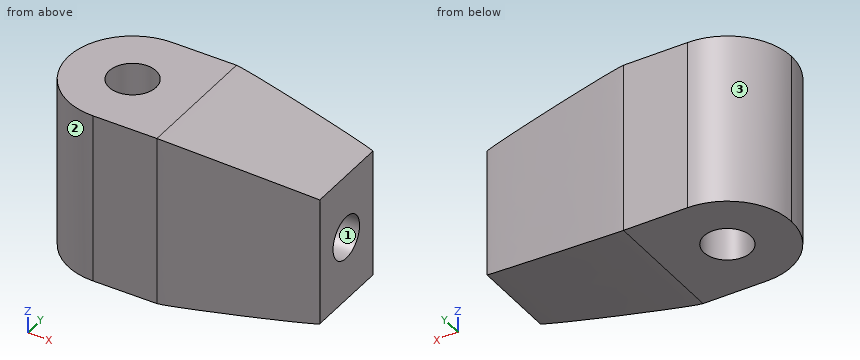
from build123d import *

# Parameters (mm, degrees)
SKETCH_1_W          = 13
SKETCH_1_H          = 8
EXTRUDE_1_DEPTH     = 6
SKETCH_2_R          = 1.1
CUT_EXTRUDE_1_DEPTH = 17.401219467
SKETCH_3_R          = 1
CUT_EXTRUDE_2_DEPTH = 8
FILLET_1_SIZE       = 1
FILLET_1_SIZE_2     = 7
FILLET_2_R          = 3


# Some blends are built 0.0001 mm under size
with BuildPart() as part:
    # 草图1 → 凸台-拉伸1 (new body)
    with BuildSketch(Plane(origin=(0, 0, 0), x_dir=(1, 0, 0), z_dir=(0, 1, 0))):
        with Locations((6.5, 4)):
            Rectangle(SKETCH_1_W, SKETCH_1_H)
    extrude(amount=EXTRUDE_1_DEPTH)

    # 草图2 → 切除-拉伸1 (cut, through all)
    with BuildSketch(Plane.XY):
        with Locations((3, 3)):
            Circle(SKETCH_2_R)
    extrude(amount=-CUT_EXTRUDE_1_DEPTH, mode=Mode.SUBTRACT)

    # 草图3 → 切除-拉伸2 (cut)
    with BuildSketch(Plane(origin=(13, 0, 0), x_dir=(0, 0, -1), z_dir=(1, 0, 0))):
        with Locations((4, 3)):
            Circle(SKETCH_3_R)
    extrude(amount=-CUT_EXTRUDE_2_DEPTH, mode=Mode.SUBTRACT)

    # 圆角1
    # a fillet whose section is not a circle: 7, 1 mm, written as the material it takes off along each edge
    with BuildSketch(Plane(origin=(13, -17.5, -8), x_dir=(0, 0, 1), z_dir=(0, 1, 0))) as fillet_1_piece_1:
        with BuildLine():
            Bezier((FILLET_1_SIZE, 0), (0, 0), (0, -FILLET_1_SIZE_2), weights=[1, 0.052631579, 1])
            Line((0, -FILLET_1_SIZE_2), (0, 0))
            Line((0, 0), (FILLET_1_SIZE, 0))
        make_face()
    extrude(amount=41, mode=Mode.SUBTRACT)
    with BuildSketch(Plane(origin=(13, 0, 17.5), x_dir=(-1, 0, 0), z_dir=(0, 0, -1))) as fillet_1_piece_2:
        with BuildLine():
            Bezier((FILLET_1_SIZE_2, 0), (0, 0), (0, FILLET_1_SIZE), weights=[1, 0.052631579, 1])
            Line((0, FILLET_1_SIZE), (0, 0))
            Line((0, 0), (FILLET_1_SIZE_2, 0))
        make_face()
    extrude(amount=43, mode=Mode.SUBTRACT)
    with BuildSketch(Plane(origin=(13, -17.5, 0), x_dir=(-1, 0, 0), z_dir=(0, 1, 0))) as fillet_1_piece_3:
        with BuildLine():
            Bezier((FILLET_1_SIZE_2, 0), (0, 0), (0, -FILLET_1_SIZE), weights=[1, 0.052631579, 1])
            Line((0, -FILLET_1_SIZE), (0, 0))
            Line((0, 0), (FILLET_1_SIZE_2, 0))
        make_face()
    extrude(amount=41, mode=Mode.SUBTRACT)
    with BuildSketch(Plane(origin=(13, 6, 17.5), x_dir=(-1, 0, 0), z_dir=(0, 0, -1))) as fillet_1_piece_4:
        with BuildLine():
            Bezier((FILLET_1_SIZE_2, 0), (0, 0), (0, -FILLET_1_SIZE), weights=[1, 0.052631579, 1])
            Line((0, -FILLET_1_SIZE), (0, 0))
            Line((0, 0), (FILLET_1_SIZE_2, 0))
        make_face()
    extrude(amount=43, mode=Mode.SUBTRACT)

    # 圆角2
    fillet_2_edges = [part.edges().sort_by_distance(p)[0] for p in [
        (0, 0, -4),
        (0, 6, -4),
    ]]
    fillet(fillet_2_edges, radius=FILLET_2_R - 0.0001)  # a hair under: the kernel refuses the full size


solid = part.part
The listing builds one solid part. Answer for the finished solid, in the listing's coordinates (mm). Face numbers are marked on the shaded views. Give positions to 0.01 mm unless a question says otherwise; leave off trailing zeros. Write each loop counter-clockwise with the first axis right and the second up, starting at its lowest first coordinate (ties: lowest second). Pieces come first, ordered by that corner, then holes.
Item 1: Flat-ended cylindrical pins translate along their axes: P1, Ø1.5, axis at x = 9, y = 4.5, coming from the +Z side; P2, Ø1.8, axis at y = 3, z = -4, coming from the +X side; P3, Ø3, axis at x = 6.5, z = -3, coming from the -Y side; P4, Ø2, axis at y = 4.5, z = -4, coming from the -X side. Find the tip coordinate at first contact, or state that the pin passes through.
Item 2: Find the intervals of material crossed by line 1 along Y through (x, z) = (3, -2.5); line 2 along Y through (x, z) = (11, -4); line 3 along X through (y, z) = (2.75, -3), in increasing order.
Item 3: Determine the mould class of the marked faces 1, 2 and 3 for opening direction Y: released by +Y, released by -Y, zero draft, split by the parting line, or undercut.
Item 4: Section B-B, the plane x = 1 is taken. Write down the section's boundary in (y, z), plus the area to 3 significant figures.
Item 5: Section A-A, the plane x = 5.5 is taken. Write down the section's boundary in (y, z), plus the area to 3 significant figures.
Completed:
1. P1: stops at z = -0.28
1. P2: stops at x = 5
1. P3: stops at y = 0
1. P4: stops at x = 0.04
2. line 1: y = 0 to 1.9, 4.1 to 6
2. line 2: y = 0.67 to 2, 4 to 5.33
2. line 3: x = 0.01 to 1.93, 4.07 to 13
3. face 1: undercut
3. face 2: released by -Y
3. face 3: released by +Y
4. outline: (0.76, -8) - (5.24, -8) - (5.24, 0) - (0.76, 0) - close
4. area: 35.8 mm2
5. outline: (0, -8) - (6, -8) - (6, 0) - (0, 0) - close; hole circle Ø2 at (3, -4)
5. area: 44.9 mm2
